Verification items for this drawing (mm, ordinates from the low corner). A direction names the side the tool comes from. Coordinates: 2 decimals unless noted, no trailing zeros. Write each loop counter-clockwise with the first axis right and the second up, starting at its lowest first coordinate (ties: lowest second). Pieces come first, ordered by that corner, then holes. Notation, with made-up numbers: (-29.5, 26.5) -> (22.5, 26.5) arc R33 ccw to (22.5, 63.5) -> close; hole circle Ø8 at (38, -29.75). An arc over 180 degrees is marked (long way). One line per item, written item: value. Start each with the question number.
1) Sectioned sample at D-D on z = 14. Enter the section's corners in (x, y) (1 decimal).
2) Scan lines: line 1 along X through (y, z) = (39, 4.5); line 2 along Y through (x, z) = (45.5, 59.5) (1 decimal); line 3 along X through (y, z) = (41.5, 58.5). Record each from-to range of solid material in increasing order. Write a range as [from, to].
3) Sectioned sample at B-B on x = 16. Give the number of separate pieces and of enclosed holes in the cut face.
4) Set-up check for the marked faces 4, 5, 6 and 7: record each of +Z, -Z, +X, -X, +Y, -Y from which the full face is reachable in a straight line by a thin tool's end or side.
5) Sectioned sample at A-A on z = 42. Enter the section's corners in (x, y) (1 decimal).
6) Gauge pin test, flat ends, axial feed: P1, Ø7, axis at x = 47, y = 31, coming from the -Z side; P2, Ø12, axis at y = 20, z = 51, coming from the +X side; P3, Ø6, axis at x = 56.5, y = 49, coming from the +Z side; P4, Ø13, axis at x = 16, y = 35, coming from the +Z side (1 decimal). Record the tip position at first contact, or that the pin passes through.
7) Draft check along Z on the marked faces 1, 2 and 3. Enter one of: +Z half, -Z half, draft (parallel to the pull), parting line (faces both ways), or undercut.
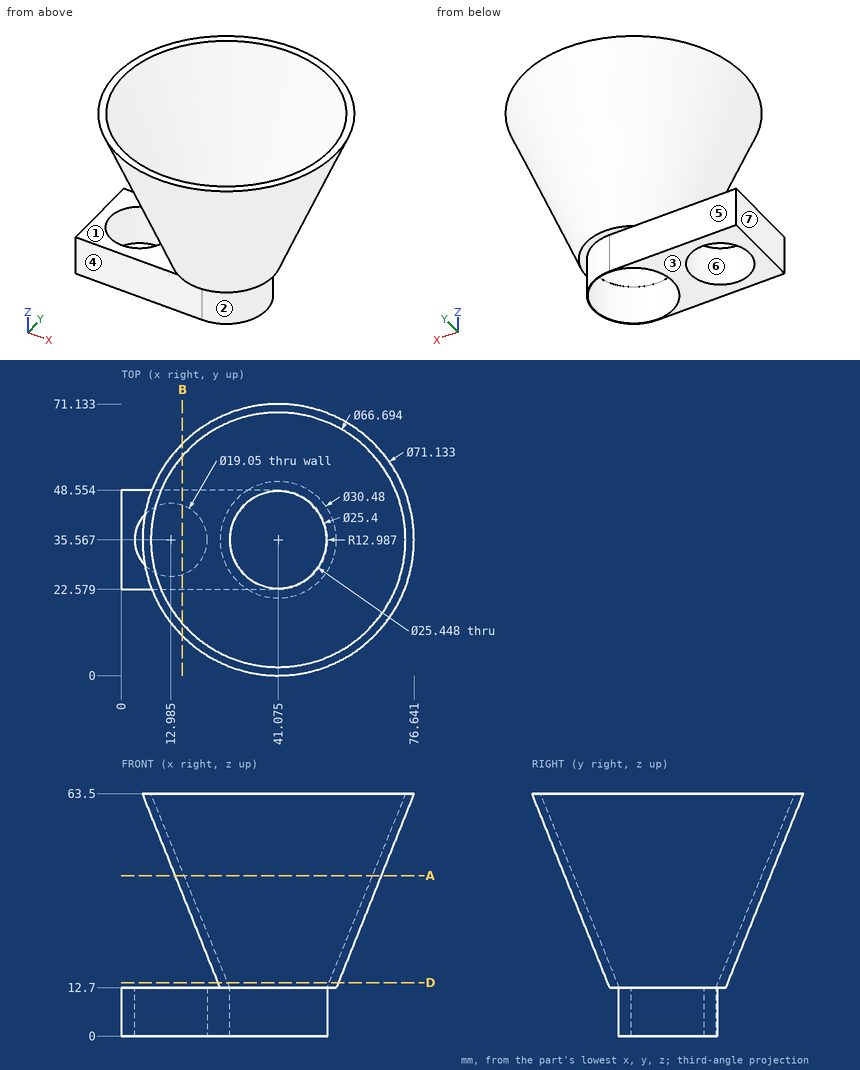
Answers:
1. outline: circle Ø31.5 at (41.1, 35.6); hole circle Ø26.5 at (41.1, 35.6)
2. line 1: x = [0, 4.1], [21.87, 28.82], [53.33, 53.6]
2. line 2: y = [1.9, 4.2], [67, 69.2]
2. line 3: x = [8.04, 10.33], [71.82, 74.11]
3. separate pieces: 3
3. enclosed holes: 0
4. face 4: -Z, +X, -X, -Y
4. face 5: -Z, +X, -X, +Y
4. face 6: -Z
4. face 7: +Z, -Z, -X, +Y, -Y
5. outline: circle Ø53.9 at (41.1, 35.6); hole circle Ø49.2 at (41.1, 35.6)
6. P1: passes through
6. P2: stops at x = 71.29
6. P3: stops at z = 39.16
6. P4: stops at z = 59.2
7. face 1: undercut
7. face 2: draft
7. face 3: -Z half
